from build123d import *

# Parameters (mm, degrees)
F2_W      = 5
F2_H      = 2
F5_W      = 5
F5_H      = 12.5
F6_DEPTH  = 5
F7_W      = 3
F7_H      = 8.5
F8_DEPTH  = 5.0010001
F9_W      = 5
F9_H      = 2
F10_DEPTH = 2
F11_R     = 2


with BuildPart() as f3:
    # F3: sweep along a path in F1
    with BuildLine(Plane.YZ) as f3_path:
        Line((4, 8), (4, 18.6544566876))
        ThreePointArc((4, 18.6544566876), (2, 20), (0, 18.6544566876))
        Line((0, 18.6544566876), (0, 0))
        Line((0, 0), (0, -18.6544566876))
        ThreePointArc((0, -18.6544566876), (2, -20), (4, -18.6544566876))
        Line((4, -18.6544566876), (4, -8))
    # F2 (on Top) → F3 (sweep)
    with BuildSketch(Plane.XY):
        Rectangle(F2_W, F2_H)
    sweep(path=f3_path.line, transition=Transition.RIGHT)

    # F5 (on face) → F6 (join)
    with BuildSketch(Plane.XZ.offset(1)):
        Rectangle(F5_W, F5_H)
    extrude(amount=F6_DEPTH)

    # F7 (on face) → F8 (cut, through all)
    with BuildSketch(Plane.YZ.offset(2.5)):
        with Locations((-2.5, 0)):
            Rectangle(F7_W, F7_H)
    extrude(amount=-F8_DEPTH, mode=Mode.SUBTRACT)

    # F9 (on face) → F10 (cut, through all)
    with BuildSketch(Plane(origin=(0, 0, -6.25), x_dir=(1, 0, 0), z_dir=(0, 0, -1))):
        with Locations((0, 2)):
            Rectangle(F9_W, F9_H)
    extrude(amount=-F10_DEPTH, mode=Mode.SUBTRACT)

    # F11
    f11_edges = [f3.edges().sort_by_distance(p)[0] for p in [
        (0, -6, 6.25),
        (0, -6, -6.25),
    ]]
    fillet(f11_edges, radius=F11_R)


solid = f3.part
The model under review builds one solid part; all positions refer to its coordinate system, in mm. A direction names the side the tool comes from. Give positions to 0.01 mm unless a question says otherwise; leave off trailing zeros. Write each loop counter-clockwise with the first axis right and the second up, starting at its lowest first coordinate (ties: lowest second). Pieces come first, ordered by that corner, then holes. Notation, with made-up numbers: M 57.5,69 L 89.5,69 A9 ccw 89.5,78 Z; hole C 71.5,-37 d10. An arc over 180 degrees is marked long. One line per question, with ' | ' between items. Start each with the question number.
Item 1: Wall thickness on line 1 (Y direction, x = 1.9, z = -15.5); line 2 (Z direction, x = -1.65, y = -3.75); line 3 (Y direction, x = -0.4, z = 0.5): over which ranges is each line inside the solid? List them lowest first. Write a range as from..to.
Item 2: We need section A-A on z = -15.5. Write out the cut boundary in (x, y).
Item 3: For pin 1 (2.5 mm diameter, centred on x = -0.5, y = -3, fed in from +Z); pin 2 (2.5 mm diameter, centred on x = 0.5, z = 0, fed in from +Y); pin 3 (1 mm diameter, centred on x = -0.5, y = 3.5, fed in from -Z), all flat-tipped, find the tip position at first contact; note any pin that passes through.
Item 4: Draft analysis for pull direction Y (two halves, no side actions). For faces 1 (the cylindrical face through (0.04, -5.43, 5.65)), 2 (the flat face through (0, -3, -5)), 3 (the flat face through (2.5, 0.8, 0.3)), state which applies: released by +Y, released by -Y, zero draft, split by the parting line, or undercut.
Item 5: We need section C-C on y = -4.75. Write out the cut boundary in (x, z), plus the area to 3 significant figures.
Item 6: For faces 4 (the flat face through (0, 4, 8)), 5 (the flat face through (0, 1, 0)), 6 (the flat face through (0, -1, -7)), list the 3-axis set-ups (+Z, -Z, +X, -X, +Y, -Y) from which the entire face can be reached by the end or side of a thin tool; tool diameter is ignored.
Item 7: We need section B-B on y = -2. Write out the cut boundary in (x, z).
Results found:
1) line 1: y = -1..1, 3..5 | line 2: z = -6.25..-4.25, 4.25..6.25 | line 3: y = -6..-4, -1..1
2) outline: M -2.5,-1 L 2.5,-1 L 2.5,1 L -2.5,1 Z; M -2.5,3 L 2.5,3 L 2.5,5 L -2.5,5 Z
3) pin 1: stops at z = 6.25 | pin 2: stops at y = 1 | pin 3: stops at z = -20.84
4) face 1: released by -Y | face 2: undercut | face 3: zero draft
5) outline: M -2.5,-6.1 L 2.5,-6.1 L 2.5,6.1 L -2.5,6.1 Z | area: 61.0 mm2
6) face 4: +X, -X, +Y | face 5: +X, -X | face 6: -Z, +X, -X
7) outline: M -2.5,4.25 L 2.5,4.25 L 2.5,6.25 L -2.5,6.25 Z
